For this review, take the finished solid that the model builds, in its own axes (mm). A direction names the side the tool comes from. Round coordinates to 2 decimals unless told otherwise and drop trailing zeros. Order: outer loops, then holes, each group sorted by start corner. A loop starts at its lowest first (then second) coordinate and runs counter-clockwise, first axis right, second up. Notation, with made-up numbers: M 58,34 L 103,34 A21 cw 103,72 Z; hole C -6.5,71 d7. An arc over 180 degrees is marked long. Write item = value, one per line. Start each with the question number.
from build123d import *

# Parameters (mm, degrees)
F0_R     = 3.0805460827
F1_DEPTH = 5


with BuildPart() as f1:
    # F0 (on Top) → F1 (new body)
    with BuildSketch(Plane.XY):
        with BuildLine():
            ThreePointArc((38.7372693115, -21.1983433866), (31.1931013311, -7.1196218248), (44.0986901689, 2.2915761904))
            ThreePointArc((44.0986901689, 2.2915761904), (37.273760147, 8.5074925195), (40.7258246034, 17.0690657747))
            ThreePointArc((40.7258246034, 17.0690657747), (25.0149250542, 19.9487370556), (25.7034571856, 35.9065186946))
            ThreePointArc((25.7034571856, 35.9065186946), (16.5883838399, 34.4461339782), (12.0470033135, 42.4831202622))
            ThreePointArc((12.0470033135, 42.4831202622), (0, 31.9952900531), (-12.0470033135, 42.4831202622))
            ThreePointArc((-12.0470033135, 42.4831202622), (-12.0206191757, 42.1068190332), (-12.0118180753, 41.729696668))
            ThreePointArc((-12.0118180753, 41.729696668), (-16.9319780047, 34.2904362337), (-25.7034571856, 35.9065186946))
            ThreePointArc((-25.7034571856, 35.9065186946), (-23.2277433364, 32.0404826351), (-22.3613630755, 27.5321815005))
            ThreePointArc((-22.3613630755, 27.5321815005), (-28.503168199, 16.9641845533), (-40.7258246034, 17.0690657747))
            ThreePointArc((-40.7258246034, 17.0690657747), (-38.0432125415, 14.1499197283), (-37.0710737614, 10.3063839463))
            ThreePointArc((-37.0710737614, 10.3063839463), (-39.0767925501, 4.9766434335), (-44.0986901689, 2.2915761904))
            ThreePointArc((-44.0986901689, 2.2915761904), (-34.8293180265, -0.8629063864), (-30.8881520208, -9.8261218116))
            ThreePointArc((-30.8881520208, -9.8261218116), (-33.040951009, -16.7351026662), (-38.7372693115, -21.1983433866))
            ThreePointArc((-38.7372693115, -21.1983433866), (-31.471625408, -22.3291562996), (-28.1275289546, -28.8778460989))
            ThreePointArc((-28.1275289546, -28.8778460989), (-28.4227133995, -31.0424462167), (-29.2867100058, -33.0489699248))
            ThreePointArc((-29.2867100058, -33.0489699248), (-15.640987417, -28.142300009), (-6.9966203098, -39.7851549832))
            ThreePointArc((-6.9966203098, -39.7851549832), (-7.14303654, -41.6667113538), (-7.5787601318, -43.5029676105))
            ThreePointArc((-7.5787601318, -43.5029676105), (0, -38.2323243404), (7.5787601318, -43.5029676105))
            ThreePointArc((7.5787601318, -43.5029676105), (13.8822360824, -28.8267602574), (29.2867100058, -33.0489699248))
            ThreePointArc((29.2867100058, -33.0489699248), (29.8912348172, -23.8374643276), (38.7372693115, -21.1983433866))
        make_face()
        with Locations((-20.6125697417, -11.9006726891)):
            Circle(F0_R, mode=Mode.SUBTRACT)
        with Locations((20.6125697417, -11.9006726891)):
            Circle(F0_R, mode=Mode.SUBTRACT)
        with BuildLine():
            ThreePointArc((7.7599617955, 15.8301915799), (14.9602642781, 9.3275112035), (17.6298602525, 0))
            ThreePointArc((17.6298602525, 0), (17.619724514, -0.5977295172), (17.5893289527, -1.1947717426))
            ThreePointArc((17.5893289527, -1.1947717426), (15.2679068439, -8.8149301263), (9.8293671572, -14.6354198373))
            ThreePointArc((9.8293671572, -14.6354198373), (0, -17.6298602525), (-9.8293671572, -14.6354198373))
            ThreePointArc((-9.8293671572, -14.6354198373), (-15.2679068439, -8.8149301263), (-17.5893289527, -1.1947717426))
            ThreePointArc((-17.5893289527, -1.1947717426), (-15.2679068439, 8.8149301263), (-7.7599617955, 15.8301915799))
            ThreePointArc((-7.7599617955, 15.8301915799), (-4.3804103986, 18.8544554654), (-3.0730313634, 23.1970698569))
            ThreePointArc((-3.0730313634, 23.1970698569), (-0.303567141, 26.9184783007), (3.1318797336, 23.8013453782))
            ThreePointArc((3.1318797336, 23.8013453782), (3.1171329225, 23.4977782372), (3.0730313634, 23.1970698569))
            ThreePointArc((3.0730313634, 23.1970698569), (4.3804103986, 18.8544554654), (7.7599617955, 15.8301915799))
        make_face(mode=Mode.SUBTRACT)
        with BuildLine():
            ThreePointArc((-22.3613630755, 27.5321815005), (-23.2277433364, 32.0404826351), (-25.7034571856, 35.9065186946))
            ThreePointArc((-25.7034571856, 35.9065186946), (-34.5242636109, 27.5321815005), (-40.7258246034, 17.0690657747))
            ThreePointArc((-40.7258246034, 17.0690657747), (-28.503168199, 16.9641845533), (-22.3613630755, 27.5321815005))
        make_face()
        with BuildLine():
            ThreePointArc((-44.0986901689, 2.2915761904), (-43.0510525562, -9.8261218116), (-38.7372693115, -21.1983433866))
            ThreePointArc((-38.7372693115, -21.1983433866), (-33.040951009, -16.7351026662), (-30.8881520208, -9.8261218116))
            ThreePointArc((-30.8881520208, -9.8261218116), (-34.8293180265, -0.8629063864), (-44.0986901689, 2.2915761904))
        make_face()
        with BuildLine():
            ThreePointArc((-29.2867100058, -33.0489699248), (-19.1595208452, -39.7851549832), (-7.5787601318, -43.5029676105))
            ThreePointArc((-7.5787601318, -43.5029676105), (-7.14303654, -41.6667113538), (-6.9966203098, -39.7851549832))
            ThreePointArc((-6.9966203098, -39.7851549832), (-15.640987417, -28.142300009), (-29.2867100058, -33.0489699248))
        make_face()
        with BuildLine():
            ThreePointArc((7.5787601318, -43.5029676105), (19.1595208452, -39.7851549832), (29.2867100058, -33.0489699248))
            ThreePointArc((29.2867100058, -33.0489699248), (13.8822360824, -28.8267602574), (7.5787601318, -43.5029676105))
        make_face()
        with BuildLine():
            ThreePointArc((38.7372693115, -21.1983433866), (42.781500191, -10.9402485099), (44.1581905885, 0))
            ThreePointArc((44.1581905885, 0), (44.1433129774, 1.1461742599), (44.0986901689, 2.2915761904))
            ThreePointArc((44.0986901689, 2.2915761904), (31.1931013311, -7.1196218248), (38.7372693115, -21.1983433866))
        make_face()
        with BuildLine():
            ThreePointArc((25.7034571856, 35.9065186946), (25.0149250542, 19.9487370556), (40.7258246034, 17.0690657747))
            ThreePointArc((40.7258246034, 17.0690657747), (34.5242636109, 27.5321815005), (25.7034571856, 35.9065186946))
        make_face()
        with BuildLine():
            ThreePointArc((-12.0470033135, 42.4831202622), (0, 31.9952900531), (12.0470033135, 42.4831202622))
            ThreePointArc((12.0470033135, 42.4831202622), (0, 44.1581905885), (-12.0470033135, 42.4831202622))
        make_face()
    extrude(amount=F1_DEPTH)


solid = f1.part
(1) Insertion check: pin 1 (3 mm diameter, centred on x = -5, z = 0.5, fed in from -Y); pin 2 (1 mm diameter, centred on x = 15, z = 3, fed in from -Y); pin 3 (3 mm diameter, centred on y = 6.5, z = 2.5, fed in from -X). Each pin has a flat end and moves straight along its axis. Give the tip position at first contact, or say it passes through.
(2) We need section C-C, the plane z = 1.8. Write out the cut boundary in (x, y), then the cut area to 3 significant figures.
(3) For faces 1 (the cylindrical face through (19.005, -39.859, 2.465)), 2 (the cylindrical face through (-4.415, 18.8, 2.465)), list the 3-axis set-ups (+Z, -Z, +X, -X, +Y, -Y) from which the entire face can be reached by the end or side of a thin tool; tool diameter is ignored.
(4) We need section A-A, the plane x = 0. Write out the cut boundary in (y, z).
(5) For line 1 along X through (y, z) = (1, 2.85); line 2 along X through (y, z) = (-11, 4.5); line 3 along X through (y, z) = (-28.5, 2.6), list the stretches that pass through material, from the lowest coordinate up.
(6) Draft analysis for pull direction Y (two halves, no side actions). For faces 3 (the cylindrical face through (29.806, -23.946, 2.465)), 4 (the cylindrical face through (-0.138, -38.233, 2.465)), 5 (the flat face through (-1, -19, 5)), state which applies: released by +Y, released by -Y, zero draft, split by the parting line, or undercut.
(7) We need section D-D, the plane y = -30. Write out the cut boundary in (x, z), then the cut area to 3 significant figures.
(8) We need section B-B, the plane y = 13. Write out the cut boundary in (x, z).
Values:
q1.pin_1 = -41.51
q1.pin_2 = -41.71
q1.pin_3 = -39.06
q2.outline = M -44.1,2.29 A44.16 ccw -38.74,-21.2 A8.08 cw -29.29,-33.05 A44.16 ccw -7.58,-43.5 A8.08 cw 7.58,-43.5 A44.16 ccw 29.29,-33.05 A8.08 cw 38.74,-21.2 A44.16 ccw 44.1,2.29 A8.08 cw 40.73,17.07 A44.16 ccw 25.7,35.91 A8.08 cw 12.05,42.48 A44.16 ccw -12.05,42.48 A8.08 cw -25.7,35.91 A44.16 ccw -40.73,17.07 A8.08 cw Z; hole C -20.61,-11.9 d6.16; hole M -7.76,15.83 A17.63 ccw long 7.76,15.83 A8.37 cw 3.07,23.2 A3.13 ccw long -3.07,23.2 A8.37 cw Z; hole C 20.61,-11.9 d6.16
q2.area = 4,570 mm²
q3.face_1 = +Z, -Z, +X, -Y
q3.face_2 = +Z, -Z
q4.outline = M -38.23,0 L -17.63,0 L -17.63,5 L -38.23,5 Z; M 26.93,0 L 44.16,0 L 44.16,5 L 26.93,5 Z
q5.line_1 = -44.15 to -17.6, 17.6 to 44.15
q5.line_2 = -42.77 to -23.56, -17.67 to -13.78, 13.78 to 17.67, 23.56 to 42.77
q5.line_3 = -28.14 to 28.14
q6.face_3 = undercut
q6.face_4 = released by -Y
q6.face_5 = zero draft
q7.outline = M -28.21,0 L 28.21,0 L 28.21,5 L -28.21,5 Z
q7.area = 282 mm²
q8.outline = M -37.53,0 L -11.91,0 L -11.91,5 L -37.53,5 Z; M 11.91,0 L 37.53,0 L 37.53,5 L 11.91,5 Z
